Can you work these out from the drawing? Everything is in mm from the part's minimum corner. Coordinates: 2 decimals unless noted, no trailing zeros. Order: outer loops, then holes, each group sorted by start corner. A loop starts at its lowest first (then second) coordinate and runs counter-clockwise, first axis right, second up. Notation, with made-up numbers: (-39, 85) -> (8, 85) arc R9 cw to (8, 93) -> close; hole circle Ø11 at (24, 43.25). An arc over 180 degrees is marked (long way). Answer in a Markdown table with one row per item.
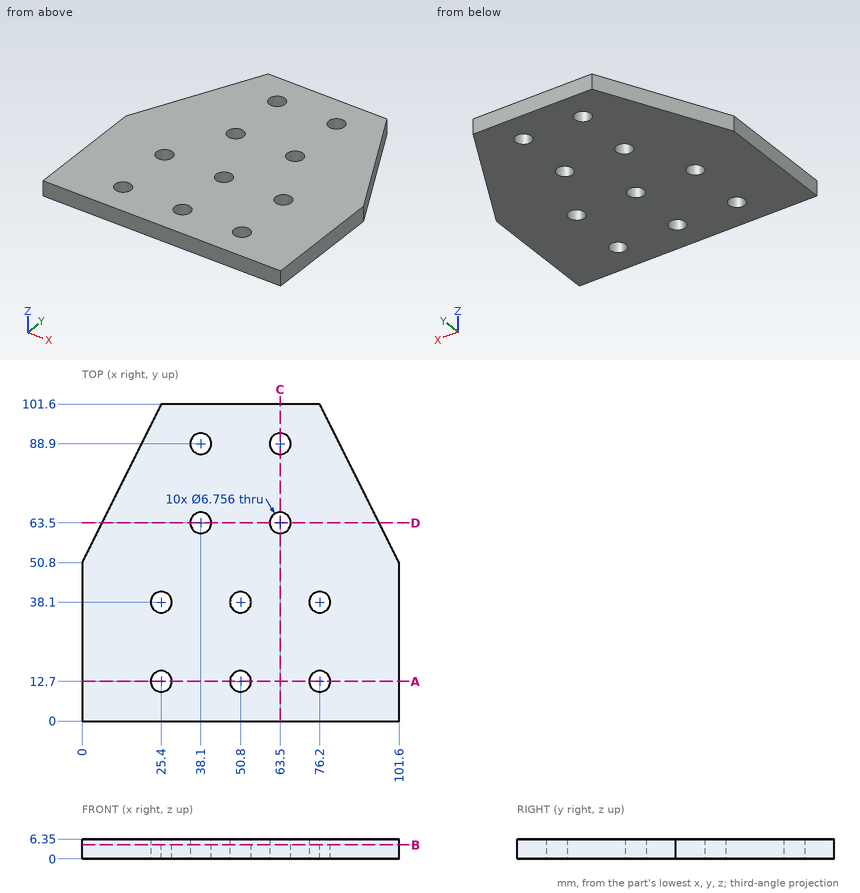
(1) Suppose I cut it at C-C (x = 63.5). Please give me the cut outline in (y, z).
Response values:
| item | result |
|---|---|
| outline | (0, 0) -> (60.12, 0) -> (60.12, 6.35) -> (0, 6.35) -> close; (66.88, 0) -> (85.52, 0) -> (85.52, 6.35) -> (66.88, 6.35) -> close; (92.28, 0) -> (101.6, 0) -> (101.6, 6.35) -> (92.28, 6.35) -> close |
(2) Suppose I cut it at D-D (y = 63.5). Please give me the cut outline in (x, z), and give its area (3 significant figures).
Response values:
| item | result |
|---|---|
| outline | (6.35, 0) -> (34.72, 0) -> (34.72, 6.35) -> (6.35, 6.35) -> close; (41.48, 0) -> (60.12, 0) -> (60.12, 6.35) -> (41.48, 6.35) -> close; (66.88, 0) -> (95.25, 0) -> (95.25, 6.35) -> (66.88, 6.35) -> close |
| area | 479 mm2 |
(3) Suppose I cut it at B-B (z = 4.5). Count the separate pieces of the cut face and the enclosed holes in it, and give its area (3 significant figures).
Response values:
| item | result |
|---|---|
| separate pieces | 1 |
| enclosed holes | 10 |
| area | 8,670 mm2 |
(4) Will this pin go through, and if not, where does the flat tip stop? pin 1 Ø2 at (y, z) = (66, 3) entering from +X.
Response values:
| item | result |
|---|---|
| pin 1 | x = 94.5 |
(5) Suppose I cut it at A-A (y = 12.7). Please give me the cut outline in (x, z).
Response values:
| item | result |
|---|---|
| outline | (0, 0) -> (22.02, 0) -> (22.02, 6.35) -> (0, 6.35) -> close; (28.78, 0) -> (47.42, 0) -> (47.42, 6.35) -> (28.78, 6.35) -> close; (54.18, 0) -> (72.82, 0) -> (72.82, 6.35) -> (54.18, 6.35) -> close; (79.58, 0) -> (101.6, 0) -> (101.6, 6.35) -> (79.58, 6.35) -> close |
(6) I need wall thicknesses on line 1 (Y direction, x = 38.1, z = 2); line 2 (Y direction, x = 76.2, z = 1.5) (1 decimal); line 3 (X direction, y = 88.9, z = 5). Which ranges of each line are inside material? Lowest first, please. Write a range as [from, to].
Response values:
| item | result |
|---|---|
| line 1 | [0, 60.12], [66.88, 85.52], [92.28, 101.6] |
| line 2 | [0, 9.3], [16.1, 34.7], [41.5, 101.6] |
| line 3 | [19.05, 34.72], [41.48, 60.12], [66.88, 82.55] |
